Answer from the drawing. Dimensions are ordinates in mm from the lowest x, y and z of the part. A direction names the side the tool comes from. Give positions to 0.01 mm unless a question says otherwise; leave off trailing zeros. Order: outer loops, then holes, each group sorted by start corner. A loop starts at its lowest first (then second) coordinate and runs counter-clockwise, first axis right, second up. Notation, with made-up numbers: M -31,-7 L -19,-7 A27 ccw -19,9 Z; hole C 84,-15 d6. An arc over 180 degrees is marked long. One line per item, written item: value.
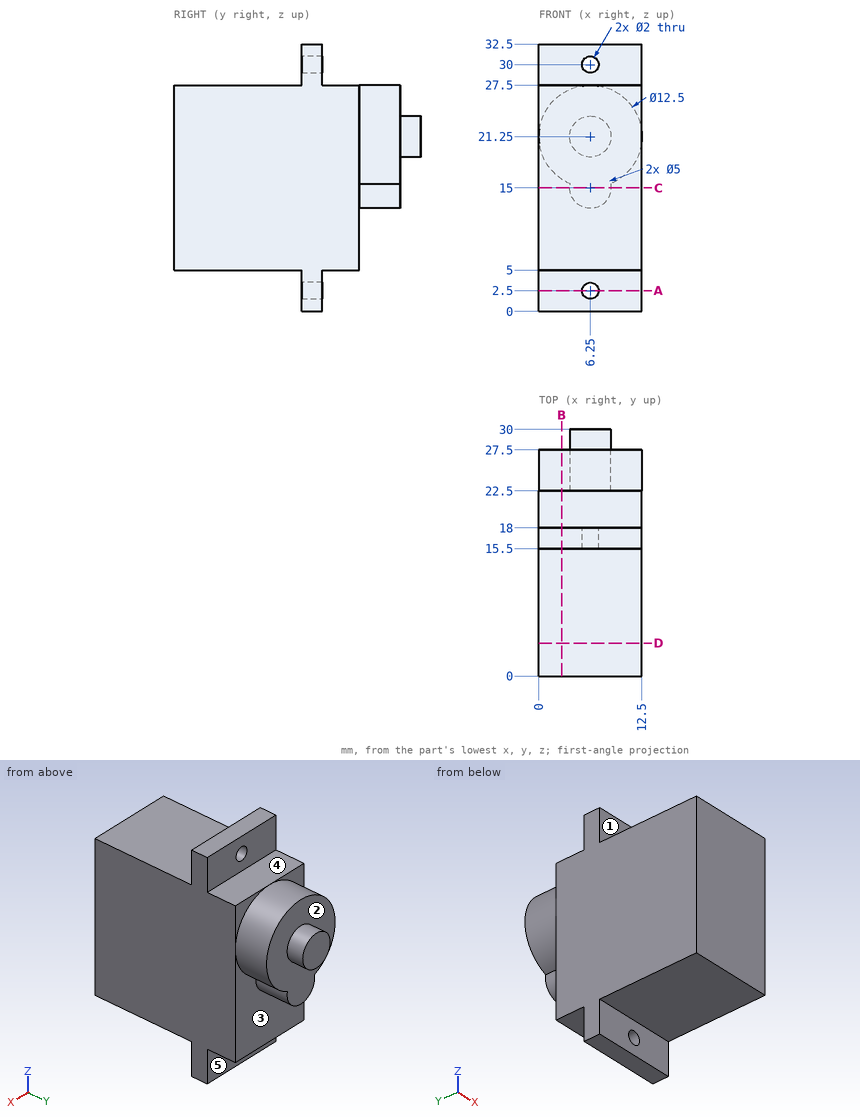
(1) Which of the six approach directions +Z, -Z, +X, -X, +Y, -Y give full straight-line access (tool end or side, diameter ignored) to the marked faces 1, 2, 3, 4 and 5?
Findings:
face 1: +Z, +X, -X, -Y
face 2: +Y
face 3: -Z, +Y
face 4: +Z, +X, -X, +Y
face 5: -Z, +X, -X, +Y
(2) Section D-D, the plane y = 4 is taken. Give the vertices of the cut face in (x, z).
Findings:
outline: M 0,5 L 12.5,5 L 12.5,27.5 L 0,27.5 Z
(3) Find the intervals of material crossed by probe 1 along X at (y, z) = (16.5, 30); probe 2 along Y at (x, z) = (9, 19); probe 3 along Y at (x, z) = (3.25, 4.5), in increasing order. Write a range as from..to.
Findings:
probe 1: x = 0..5.25, 7.25..12.5
probe 2: y = 0..27.5
probe 3: y = 15.5..18
(4) Section B-B, the plane x = 2.75 is taken. Give the vertices of the cut face in (y, z).
Findings:
outline: M 0,5 L 15.5,5 L 15.5,0 L 18,0 L 18,5 L 22.5,5 L 22.5,16.07 L 27.5,16.07 L 27.5,26.43 L 22.5,26.43 L 22.5,27.5 L 18,27.5 L 18,32.5 L 15.5,32.5 L 15.5,27.5 L 0,27.5 Z
(5) Given P1, Ø3.5, axis at x = 6.5, y = 20, coming from the -Z side; P2, Ø5.5, axis at x = 9, z = 30.5, coming from the -Y side; P3, Ø2.5, axis at x = 4.5, z = 3.5, coming from the +Y side, each flat-ended and moving along its own axis, determine where each tip first touches the part or whether it passes through.
Findings:
P1: stops at z = 5
P2: stops at y = 15.5
P3: stops at y = 18
(6) Section A-A, the plane z = 2.5 is taken. Give the vertices of the cut face in (x, y), then the cut area to 4 significant figures.
Findings:
outline: M 0,15.5 L 5.25,15.5 L 5.25,18 L 0,18 Z; M 7.25,15.5 L 12.5,15.5 L 12.5,18 L 7.25,18 Z
area: 26.25 mm^2
(7) Section C-C, the plane z = 15 is taken. Give the vertices of the cut face in (x, y), then the cut area to 3 significant figures.
Findings:
outline: M 0,0 L 12.5,0 L 12.5,22.5 L 8.75,22.5 L 8.75,27.5 L 3.75,27.5 L 3.75,22.5 L 0,22.5 Z
area: 306 mm^2
